from build123d import *

# Parameters (mm, degrees)
SKETCH1_R           = 20
SKETCH1_W           = 250
SKETCH1_H           = 15
BOSS_EXTRUDE1_DEPTH = 10
CUT_EXTRUDE1_DEPTH  = 127.984250992
FILLET1_R           = 10
CUT_EXTRUDE2_DEPTH  = 127.984250992
SKETCH6_R           = 2.5
CUT_EXTRUDE3_DEPTH  = 129.379320765
SKETCH7_R           = 2.5
CUT_EXTRUDE4_DEPTH  = 129.379320772


with BuildPart() as part:
    # Sketch1 → Boss-Extrude1 (new body)
    with BuildSketch(Plane(origin=(0, 0, 0), x_dir=(1, 0, 0), z_dir=(0, 1, 0))):
        Circle(SKETCH1_R)
        Rectangle(SKETCH1_W, SKETCH1_H)
    extrude(amount=BOSS_EXTRUDE1_DEPTH)

    # Sketch2 → Cut-Extrude1 (cut, through all)
    with BuildSketch(Plane(origin=(0, 10, 0), x_dir=(1, 0, 0), z_dir=(0, 1, 0))):
        with BuildLine():
            Line((-5, 4.898979486), (-5, -4.898979486))
            ThreePointArc((-5, -4.898979486), (0, -7), (5, -4.898979486))
            Line((5, -4.898979486), (5, 4.898979486))
            ThreePointArc((5, 4.898979486), (0, 7), (-5, 4.898979486))
        make_face()
    extrude(amount=-CUT_EXTRUDE1_DEPTH, mode=Mode.SUBTRACT)

    # Fillet1
    fillet1_edges = [part.edges().sort_by_distance(p)[0] for p in [
        (-18.540496218, 5, -7.5),
        (18.540496218, 5, -7.5),
        (-18.540496218, 5, 7.5),
        (18.540496218, 5, 7.5),
    ]]
    fillet(fillet1_edges, radius=FILLET1_R)

    # Sketch4 → Cut-Extrude2 (cut, through all)
    with BuildSketch(Plane(origin=(0, 10, 0), x_dir=(1, 0, 0), z_dir=(0, 1, 0))):
        with BuildLine():
            Line((-61.5, 3.5), (-58.5, 3.5))
            ThreePointArc((-58.5, 3.5), (-55, 0), (-58.5, -3.5))
            Line((-58.5, -3.5), (-61.5, -3.5))
            ThreePointArc((-61.5, -3.5), (-65, 0), (-61.5, 3.5))
        make_face()
        with BuildLine():
            Line((58.5, 3.5), (61.5, 3.5))
            ThreePointArc((61.5, 3.5), (65, 0), (61.5, -3.5))
            Line((61.5, -3.5), (58.5, -3.5))
            ThreePointArc((58.5, -3.5), (55, 0), (58.5, 3.5))
        make_face()
    extrude(amount=-CUT_EXTRUDE2_DEPTH, mode=Mode.SUBTRACT)

    # Sketch6 → Cut-Extrude3 (cut, through all)
    with BuildSketch(Plane.XY.offset(7.5)):
        with Locations((-60, 5)):
            Circle(SKETCH6_R)
    extrude(amount=-CUT_EXTRUDE3_DEPTH, mode=Mode.SUBTRACT)

    # Sketch7 → Cut-Extrude4 (cut, through all)
    with BuildSketch(Plane.XY.offset(7.5)):
        with Locations((60, 5)):
            Circle(SKETCH7_R)
    extrude(amount=-CUT_EXTRUDE4_DEPTH, mode=Mode.SUBTRACT)


solid = part.part
Design review of the part built by this model. Coordinates are the model's own, in mm. A direction names the side the tool comes from. Round coordinates to 2 decimals unless told otherwise and drop trailing zeros. Write each loop counter-clockwise with the first axis right and the second up, starting at its lowest first coordinate (ties: lowest second). Pieces come first, ordered by that corner, then holes. Notation, with made-up numbers: (42, 49) -> (49, 49) arc R23 ccw to (49, 78) -> close; hole circle Ø1 at (-38, 65.5). An arc over 180 degrees is marked (long way). One line per question, with ' | ' between items.
(1) Take a section at C-C, the plane x = -92. State the section outline as (y, z) points.
Result sheet:
outline: (0, -7.5) -> (10, -7.5) -> (10, 7.5) -> (0, 7.5) -> close
(2) Wall thickness on line 1 (X direction, y = 5, z = -4.5); line 2 (X direction, y = 5, z = 5); line 3 (X direction, y = 8.25, z = -4.5): over which ranges is each line inside the solid? List them lowest first. Write a range as [from, to].
Result sheet:
line 1: [-125, -62.5], [-57.5, -5], [5, 57.5], [62.5, 125] | line 2: [-125, -62.5], [-57.5, -4.9], [4.9, 57.5], [62.5, 125] | line 3: [-125, -5], [5, 125]
(3) Insertion check: P1, Ø4.5, axis at x = -60, y = 5, coming from the +Z side; P2, Ø1.5, axis at x = -65.5, z = 7, coming from the -Y side; P3, Ø2.5, axis at x = 59.5, y = 8.5, coming from the +Z side; P4, Ø2, axis at y = 1.5, z = 11.5, coming from the +X side. Each pin has a flat end and moves straight along its axis. Give the tip position at first contact, or say it passes through.
Result sheet:
P1: through | P2: y = 0 | P3: z = 7.5 | P4: x = 17.23
(4) Take a section at D-D, the plane z = -16. State the section outline as (x, y) points.
Result sheet:
outline: (-12, 0) -> (12, 0) -> (12, 10) -> (-12, 10) -> close
(5) Draft analysis for pull direction Z (two halves, no side actions). For faces 4 (the cylindrical face through (62.31, 4.04, 5.46)), 5 (the cylindrical face through (-19.744, 5.07, -8.633)), 6 (the cylindrical face through (0, 5, -7)), 7 (the flat face through (-75, 5, 7.5)), state which applies: released by +Z, released by -Z, zero draft, split by the parting line, or undercut.
Result sheet:
face 4: zero draft | face 5: released by -Z | face 6: undercut | face 7: released by +Z
(6) Machinability: for faces 1 (the cylindrical face through (65, 5, 0)), 2 (the flat face through (74, 5, 7.5)), 3 (the flat face through (-75, 5, -7.5)), which of the approach directions +Z, -Z, +X, -X, +Y, -Y give a long, thin tool a straight path to every point of the face, cutting with its end or side? Answer none if there is none.
Result sheet:
face 1: +Y, -Y | face 2: +Z, +X, +Y, -Y | face 3: -Z, -X, +Y, -Y
(7) Take a section at B-B, the plane z = 1. State the section outline as (x, y) points.
Result sheet:
outline: (-125, 0) -> (-64.85, 0) -> (-64.85, 10) -> (-125, 10) -> close; (-55.15, 0) -> (-5, 0) -> (-5, 10) -> (-55.15, 10) -> close; (5, 0) -> (55.15, 0) -> (55.15, 10) -> (5, 10) -> close; (64.85, 0) -> (125, 0) -> (125, 10) -> (64.85, 10) -> close
(8) Take a section at A-A, the plane y = 5. State how many separate pieces and enclosed holes the cut face has, and give its area (3 significant figures).
Result sheet:
separate pieces: 3 | enclosed holes: 1 | area: 4,110 mm2
